Part model, mm, in its own coordinate system. Coordinates: 2 decimals unless noted, no trailing zeros. Loops run counter-clockwise (first coordinate to the right, second up) from the corner with the lowest first, then second, coordinate; pieces in that order, holes last. Notation, with made-up numbers: M 21,76 L 80,76 A21 ccw 80,99 Z; hole C -11,-2.5 d7. An arc over 180 degrees is marked long. Answer as CSV lines item,"result". Start each with the question number.
from build123d import *

# Parameters (mm, degrees)
SKETCH1_W           = 76.2
SKETCH1_H           = 25.4
SKETCH1_R           = 3.175
BOSS_EXTRUDE1_DEPTH = 25.4
SKETCH2_R           = 6.35
CUT_EXTRUDE1_DEPTH  = 85.242269675
SCALE1_SCALE        = 1.5
SCALE2_SCALE        = 0.67


with BuildPart() as part:
    # Sketch1 → Boss-Extrude1 (new body)
    with BuildSketch(Plane.XY):
        with Locations((-38.1, 12.7)):
            Rectangle(SKETCH1_W, SKETCH1_H)
        with Locations((-38.1, 12.7)):
            Circle(SKETCH1_R, mode=Mode.SUBTRACT)
    extrude(amount=BOSS_EXTRUDE1_DEPTH)

    # Sketch2 → Cut-Extrude1 (cut, through all)
    with BuildSketch(Plane(origin=(0, 0, 0), x_dir=(0, 0, -1), z_dir=(1, 0, 0))):
        with Locations((-12.7, 12.7)):
            Circle(SKETCH2_R)
    extrude(amount=-CUT_EXTRUDE1_DEPTH, mode=Mode.SUBTRACT)


with BuildPart() as part_1:
    # Scale1: scaled about (-38.100000058, 12.700000154, 12.700000148)
    add(part.part.scale(SCALE1_SCALE).moved(Location((19.050000029, -6.350000077, -6.350000074))))


with BuildPart() as part_2:
    # Scale2: scaled about (-38.100000058, 12.700000155, 12.700000148)
    add(part_1.part.scale(SCALE2_SCALE).moved(Location((-12.573000019, 4.191000051, 4.191000049))))


solid = part_2.part
Q1. Slice it at B-B, the plane y = 12.7. Write the cut outline in (x, z).
Q2. Wall check: L1, parallel to X at y = 12.7, z = 19.5; L2, parallel to Y at x = -38.1, z = 23.25; L3, parallel to Y at x = -35, z = 12.7. Give the ranges that are in metal, low to high.
Q3. Slice it at C-C, the plane y = 17.75. Write the cut outline in (x, z).
Q4. Two-plate mould, pull along X, no slides. Class faces 1 (the face through (-76.39, 9.7, 6.8)), 2 (the face through (-35.15, 11.48, 3.5)), 3 (the face through (-39, 7, 25.463)): +X half, -X half, draft (parallel to the pull), parting line (faces both ways), or undercut.
Q5. Slice it at A-A, the plane z = 12.7. Write the cut outline in (x, y).
Q6. Slice it at D-D, the plane x = -29. Write the cut outline in (y, z), and give its area (3 significant figures).
Solved:
1,outline,"M -76.39,-0.06 L -41.29,-0.06 L -41.29,6.32 L -76.39,6.32 Z; M -76.39,19.08 L -41.29,19.08 L -41.29,25.46 L -76.39,25.46 Z; M -34.91,-0.06 L 0.19,-0.06 L 0.19,6.32 L -34.91,6.32 Z; M -34.91,19.08 L 0.19,19.08 L 0.19,25.46 L -34.91,25.46 Z"
2,L1,"x = -76.39 to -41.29, -34.91 to 0.19"
2,L2,"y = -0.06 to 9.51, 15.89 to 25.46"
2,L3,"y = -0.06 to 6.32, 19.08 to 25.46"
3,outline,"M -76.39,-0.06 L 0.19,-0.06 L 0.19,8.8 L -76.39,8.8 Z; M -76.39,16.6 L 0.19,16.6 L 0.19,25.46 L -76.39,25.46 Z"
4,face 1,"-X half"
4,face 2,"undercut"
4,face 3,"draft"
5,outline,"M -76.39,-0.06 L 0.19,-0.06 L 0.19,6.32 L -76.39,6.32 Z; M -76.39,19.08 L 0.19,19.08 L 0.19,25.46 L -76.39,25.46 Z"
6,outline,"M -0.06,-0.06 L 25.46,-0.06 L 25.46,25.46 L -0.06,25.46 Z; hole C 12.7,12.7 d12.76"
6,area,"524 mm2"
